Job drawing, mm, ordinate dimensions from the low corner. One solid piece. A direction names the side the tool comes from. Give positions to 0.01 mm unless a question says otherwise; leave off trailing zeros. Order: outer loops, then holes, each group sorted by start corner. A loop starts at its lowest first (then second) coordinate and runs counter-clockwise, first axis right, second up.
1. Slice it at C-C on z = 4. List the corners of the cut face in (x, y), and give its area (3 significant figures).
2. Drop flat-ended pins along their axis: pin 1 Ø8.5 at (y, z) = (19.5, 53) entering from -X; pin 2 Ø19 at (y, z) = (15, 54.5) entering from +X; pin 3 Ø11 at (x, y) = (53, 21.5) entering from +Z. Give the stop position or say it passes through.
3. Mould opens along X. For the marked faces 1, 2, 3 and 4 say: +X half, -X half, draft (parallel to the pull), parting line (faces both ways), or undercut.
4. Slice it at B-B on y = 13.5. List the corners of the cut face in (x, z), and give its area (3 significant figures).
5. Probe line 1 (Z direction, x = 37.5, y = 20); line 2 (X direction, y = 20, z = 4.5); line 3 (X direction, y = 22.5, z = 25). List the from-to ranges inside material, lowest first.
6. Which spindle directions (+Z, -Z, +X, -X, +Y, -Y) get a long thin tool onto all of the face, cutting with end or side? Do the marked faces 5, 6 and 7. Say none if no direction does.
7. Slice it at A-A on x = 55. List the corners of the cut face in (y, z), and give its area (3 significant figures).
8. Slice it at D-D on x = 22. List the corners of the cut face in (y, z).
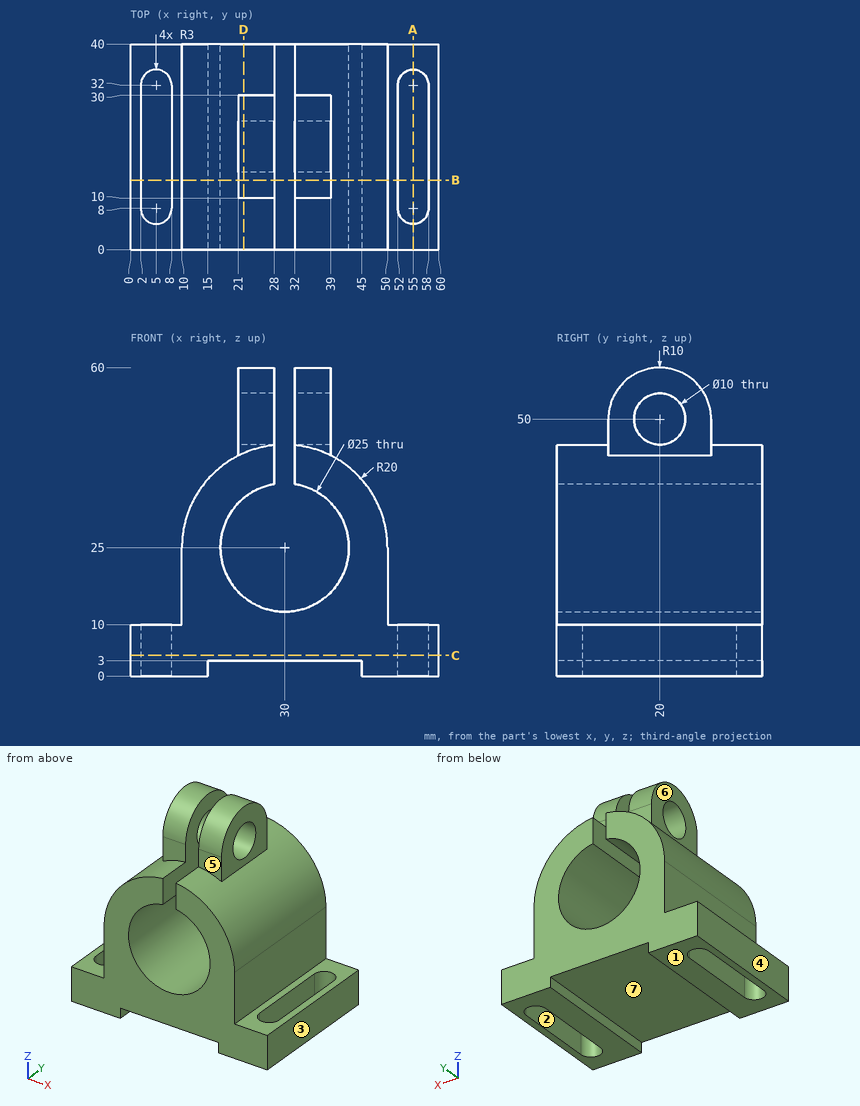
Data:
1. outline: (0, 0) - (60, 0) - (60, 40) - (0, 40) - close; hole (2, 8) arc R3 ccw to (8, 8) - (8, 32) arc R3 ccw to (2, 32) - close; hole (52, 8) arc R3 ccw to (58, 8) - (58, 32) arc R3 ccw to (52, 32) - close
1. area: 2,060 mm2
2. pin 1: stops at x = 21
2. pin 2: stops at x = 39
2. pin 3: stops at z = 34.68
3. face 1: draft
3. face 2: undercut
3. face 3: +X half
3. face 4: -X half
4. outline: (0, 0) - (2, 0) - (2, 10) - (0, 10) - close; (8, 0) - (15, 0) - (15, 3) - (45, 3) - (45, 0) - (52, 0) - (52, 10) - (50, 10) - (50, 25) arc R20 ccw to (39, 42.86) - (39, 57.6) - (32, 57.6) - (32, 37.34) arc R12.5 cw (long way) to (28, 37.34) - (28, 57.6) - (21, 57.6) - (21, 42.86) arc R20 ccw to (10, 25) - (10, 10) - (8, 10) - close; (58, 0) - (60, 0) - (60, 10) - (58, 10) - close
4. area: 1,290 mm2
5. line 1: z = 3 to 15, 35 to 45, 55 to 60
5. line 2: x = 0 to 2, 8 to 52, 58 to 60
5. line 3: x = 10 to 17.5, 42.5 to 50
6. face 5: +Z, +X, -Y
6. face 6: +Z, -X, +Y, -Y
6. face 7: -Z, +Y, -Y
7. outline: (0, 0) - (5, 0) - (5, 10) - (0, 10) - close; (35, 0) - (40, 0) - (40, 10) - (35, 10) - close
7. area: 100 mm2
8. outline: (0, 3) - (40, 3) - (40, 15.4) - (0, 15.4) - close; (0, 34.6) - (40, 34.6) - (40, 43.33) - (30, 43.33) - (30, 50) arc R10 ccw to (10, 50) - (10, 43.33) - (0, 43.33) - close; hole circle Ø10 at (20, 50)
